Part print with two shaded views. Sizes in mm from the minimum x, y, z corner. Give positions to 0.01 mm unless a question says otherwise; leave off trailing zeros. Order: outer loops, then holes, each group sorted by start corner. A loop starts at its lowest first (then second) coordinate and runs counter-clockwise, first axis right, second up. Notation, with made-up numbers: (4, 23.25) -> (11, 23.25) arc R16 ccw to (11, 31.25) -> close; hole circle Ø7 at (37.5, -28.75). An arc over 180 degrees is marked (long way). Write item = value, one per line. Start each with the question number.
Item 1: Band-saw the part on C-C on z = 47. Write the cut outline in (x, y), plus the area to 3 significant figures.
Item 2: Drill centre lines: line 1 along Z through (x, y) = (50, 57.5); line 2 along X through (y, z) = (87, 46); line 3 along X through (y, z) = (11.5, 39). Where is each one in solid material? Low to high.
Item 3: Band-saw the part on D-D on z = 11. Write the cut outline in (x, y).
Item 4: Band-saw the part on A-A on x = 50. Write the cut outline in (y, z).
Item 5: Pull direction X, two halves, no side cores. Call the marked faces 1, 2, 3 and 4: +X half, -X half, draft (parallel to the pull), parting line (faces both ways), or undercut.
Item 6: Band-saw the part on B-B on y = 77. Write the cut outline in (x, z), plus the area to 3 significant figures.
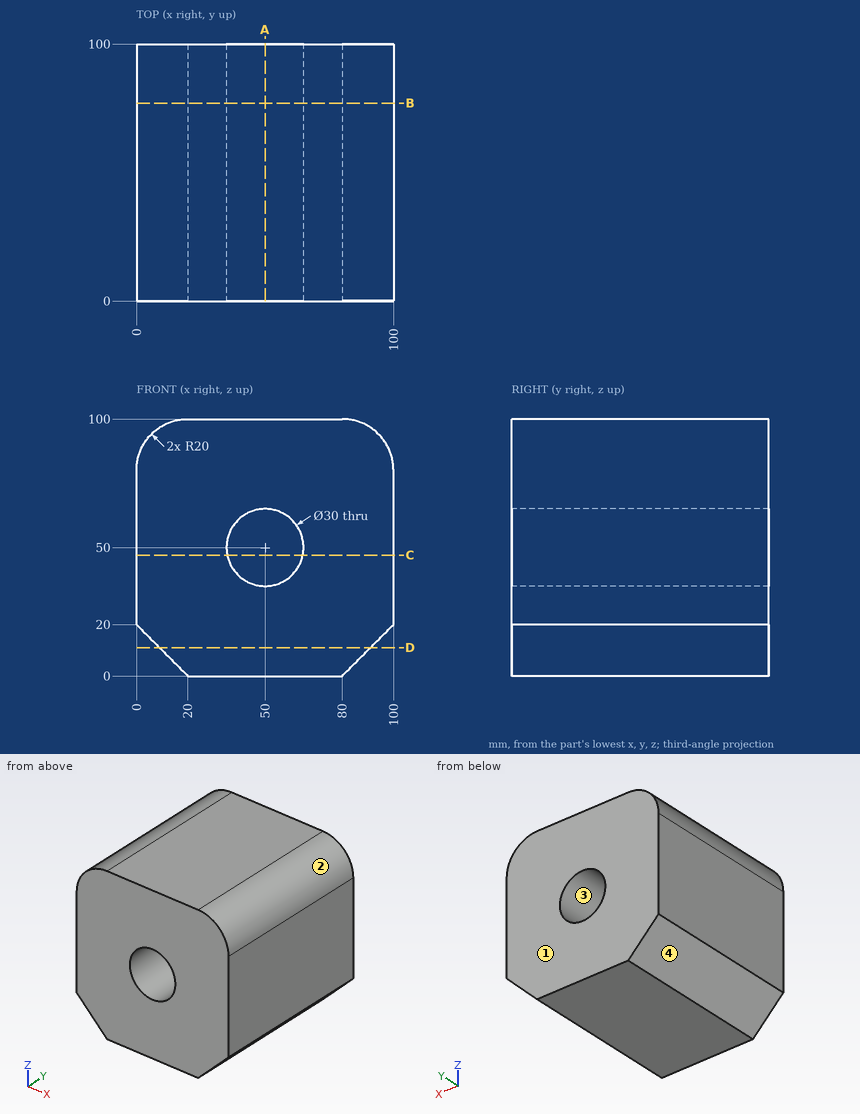
Values found:
q1.outline = (0, 0) -> (35.3, 0) -> (35.3, 100) -> (0, 100) -> close; (64.7, 0) -> (100, 0) -> (100, 100) -> (64.7, 100) -> close
q1.area = 7,060 mm^2
q2.line_1 = 0 to 35, 65 to 100
q2.line_2 = 0 to 35.54, 64.46 to 100
q2.line_3 = 0 to 39.8, 60.2 to 100
q3.outline = (9, 0) -> (91, 0) -> (91, 100) -> (9, 100) -> close
q4.outline = (0, 0) -> (100, 0) -> (100, 35) -> (0, 35) -> close; (0, 65) -> (100, 65) -> (100, 100) -> (0, 100) -> close
q5.face_1 = draft
q5.face_2 = +X half
q5.face_3 = undercut
q5.face_4 = -X half
q6.outline = (0, 20) -> (20, 0) -> (80, 0) -> (100, 20) -> (100, 80) arc R20 ccw to (80, 100) -> (20, 100) arc R20 ccw to (0, 80) -> close; hole circle Ø30 at (50, 50)
q6.area = 8,720 mm^2
